Source: three-view drawing plus pictorial views. Frame: mm from the lowest corner of the part. Round coordinates to 2 decimals unless told otherwise and drop trailing zeros. Loops run counter-clockwise (first coordinate to the right, second up) from the corner with the lowest first, then second, coordinate; pieces in that order, holes last. Notation, with made-up numbers: (-14, -24) -> (6, -24) arc R18 cw to (6, -4) -> close; hole circle Ø7 at (33, -34). An arc over 180 degrees is marked (long way). Answer in a Markdown table with one row per item.
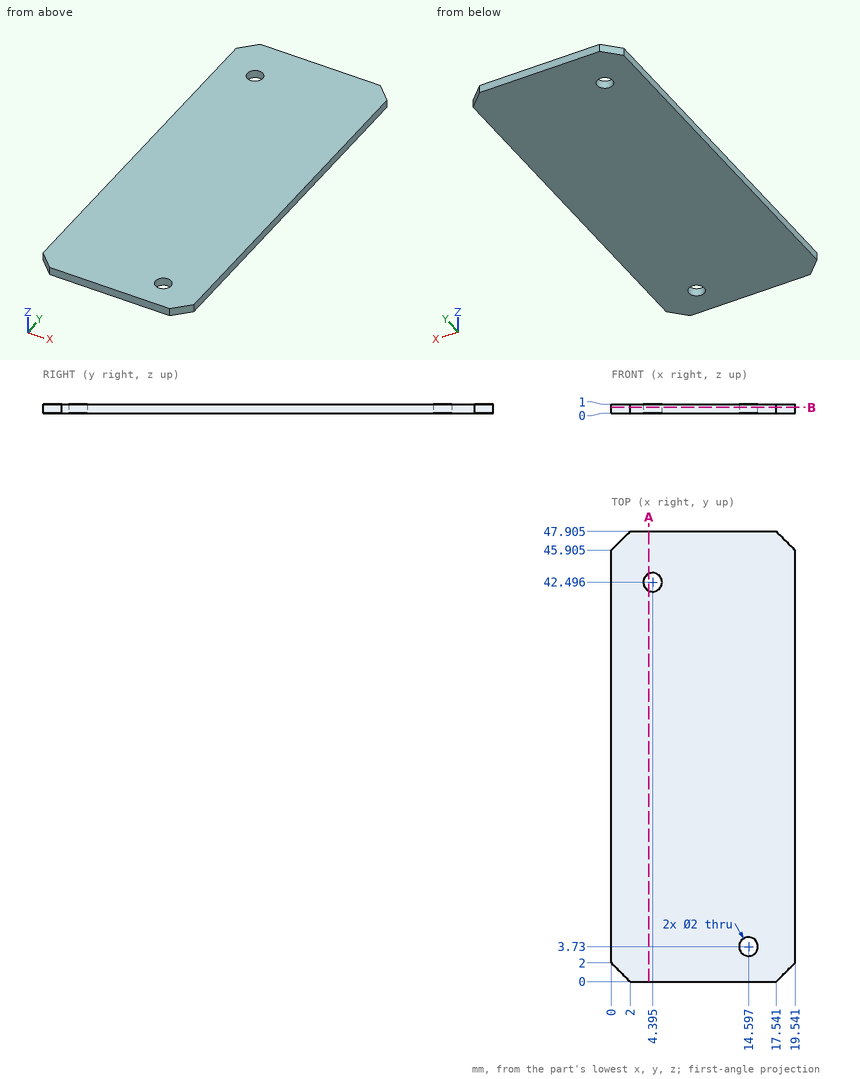
Item 1: Cut plane B-B (z = 0.65). Output: boundary loops of the cut face in (x, y) (1 decimal).
Answer:
| item | result |
|---|---|
| outline | (0, 2) -> (2, 0) -> (17.5, 0) -> (19.5, 2) -> (19.5, 45.9) -> (17.5, 47.9) -> (2, 47.9) -> (0, 45.9) -> close; hole circle Ø2 at (4.4, 42.5); hole circle Ø2 at (14.6, 3.7) |
Item 2: Line query: probe 1 along Y at (x, z) = (4.75, 0.45) (1 decimal); probe 2 along Y at (x, z) = (13.75, 0.6) (1 decimal); probe 3 along Y at (x, z) = (18.5, 0.55) (1 decimal). Output: solid intervals per line, ascending. Write a range as [from, to].
Answer:
| item | result |
|---|---|
| probe 1 | y = [0, 41.6], [43.4, 47.9] |
| probe 2 | y = [0, 3.2], [4.3, 47.9] |
| probe 3 | y = [1, 46.9] |
Item 3: Pin query (flat end, axial travel): pin 1 Ø1.2 at (x, y) = (4.39, 42.5) entering from +Z. Return the tip coordinate at first contact, or that it passes through.
Answer:
| item | result |
|---|---|
| pin 1 | passes through |
Item 4: Cut plane A-A (x = 4). Output: boundary loops of the cut face in (y, z) (1 decimal).
Answer:
| item | result |
|---|---|
| outline | (0, 0) -> (41.6, 0) -> (41.6, 1) -> (0, 1) -> close; (43.4, 0) -> (47.9, 0) -> (47.9, 1) -> (43.4, 1) -> close |
